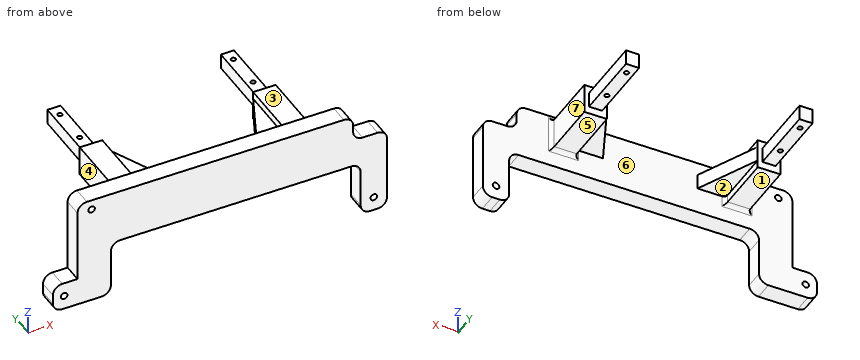
```python
from build123d import *

# Parameters (mm, degrees)
SKETCH1_R           = 1.75
BOSS_EXTRUDE1_DEPTH = 10
SKETCH3_W           = 7
SKETCH3_H           = 8
BOSS_EXTRUDE3_DEPTH = 70
CUT_EXTRUDE1_REACH  = 183.843
SKETCH4_R           = 1.25
SKETCH5_W           = 12
SKETCH5_H           = 16
BOSS_EXTRUDE4_DEPTH = 32.5
FILLET4_R           = 2
RIB1_REACH          = 184.852
SKETCH6_WALL_W      = 403.497752534
SKETCH6_WALL_H      = 8


with BuildPart() as part:
    # Sketch1 → Boss-Extrude1 (new body)
    with BuildSketch(Plane(origin=(0, 0, 0), x_dir=(1, 0, 0), z_dir=(0, 1, 0))):
        with BuildLine():
            Line((-7.5, -0.4), (-7.5, 38.6))
            Line((-7.5, 38.6), (-15.61, 38.6))
            ThreePointArc((-15.61, 38.6), (-19.145533906, 40.064466094), (-20.61, 43.6))
            Line((-20.61, 43.6), (-20.61, 48.6))
            ThreePointArc((-20.61, 48.6), (-19.145533906, 52.135533906), (-15.61, 53.6))
            Line((-15.61, 53.6), (5.26, 53.6))
            ThreePointArc((5.26, 53.6), (8.795533906, 52.135533906), (10.26, 48.6))
            Line((10.26, 48.6), (10.26, 28.6))
            ThreePointArc((10.26, 28.6), (11.724466094, 25.064466094), (15.26, 23.6))
            Line((15.26, 23.6), (138.26, 23.6))
            ThreePointArc((138.26, 23.6), (141.795533906, 25.064466094), (143.26, 28.6))
            Line((143.26, 28.6), (143.26, 48.6))
            ThreePointArc((143.26, 48.6), (144.724466094, 52.135533906), (148.26, 53.6))
            Line((148.26, 53.6), (152.26, 53.6))
            ThreePointArc((152.26, 53.6), (155.795533906, 52.135533906), (157.26, 48.6))
            Line((157.26, 48.6), (157.26, 13.6))
            ThreePointArc((157.26, 13.6), (155.795533906, 10.064466094), (152.26, 8.6))
            Line((152.26, 8.6), (144.26, 8.6))
            ThreePointArc((144.26, 8.6), (140.724466094, 7.135533906), (139.26, 3.6))
            Line((139.26, 3.6), (139.26, -0.4))
            ThreePointArc((139.26, -0.4), (137.795533906, -3.935533906), (134.26, -5.4))
            Line((134.26, -5.4), (-2.5, -5.4))
            ThreePointArc((-2.5, -5.4), (-6.035533906, -3.935533906), (-7.5, -0.4))
        make_face()
        with Locations(Location((0, 0, 0), (0, 0, 270))):
            Circle(SKETCH1_R, mode=Mode.SUBTRACT)
        with Locations(Location((-14.61, 46.1, 0), (0, 0, 270))):
            Circle(SKETCH1_R, mode=Mode.SUBTRACT)
        with Locations(Location((150.26, 46.1, 0), (0, 0, 270))):
            Circle(SKETCH1_R, mode=Mode.SUBTRACT)
    extrude(amount=BOSS_EXTRUDE1_DEPTH)

    # Sketch3 → Boss-Extrude3 (add)
    with BuildSketch(Plane(origin=(0, 10, 0), x_dir=(1, 0, 0), z_dir=(0, 1, 0))):
        with Locations((22, 5.6)):
            Rectangle(SKETCH3_W, SKETCH3_H)
        with Locations((114.32, 5.6)):
            Rectangle(SKETCH3_W, SKETCH3_H)
    extrude(amount=BOSS_EXTRUDE3_DEPTH)

    # Sketch4 → Cut-Extrude1 (cut, up to next)
    with BuildSketch(Plane(origin=(0, 0, -9.6), x_dir=(-1, 0, 0), z_dir=(0, 0, -1)), mode=Mode.PRIVATE) as cut_extrude1_sk1:
        with Locations((-22, 74)):
            Circle(SKETCH4_R)
    cut_extrude1_tool1 = extrude(cut_extrude1_sk1.sketch, amount=-CUT_EXTRUDE1_REACH, mode=Mode.PRIVATE) & part.part
    # Sketch4 → Cut-Extrude1 (cut, up to next)
    with BuildSketch(Plane(origin=(0, 0, -9.6), x_dir=(-1, 0, 0), z_dir=(0, 0, -1)), mode=Mode.PRIVATE) as cut_extrude1_sk2:
        with Locations((-22, 54)):
            Circle(SKETCH4_R)
    cut_extrude1_tool2 = extrude(cut_extrude1_sk2.sketch, amount=-CUT_EXTRUDE1_REACH, mode=Mode.PRIVATE) & part.part
    # Sketch4 → Cut-Extrude1 (cut, up to next)
    with BuildSketch(Plane(origin=(0, 0, -9.6), x_dir=(-1, 0, 0), z_dir=(0, 0, -1)), mode=Mode.PRIVATE) as cut_extrude1_sk3:
        with Locations((-114.32, 54)):
            Circle(SKETCH4_R)
    cut_extrude1_tool3 = extrude(cut_extrude1_sk3.sketch, amount=-CUT_EXTRUDE1_REACH, mode=Mode.PRIVATE) & part.part
    # Sketch4 → Cut-Extrude1 (cut, up to next)
    with BuildSketch(Plane(origin=(0, 0, -9.6), x_dir=(-1, 0, 0), z_dir=(0, 0, -1)), mode=Mode.PRIVATE) as cut_extrude1_sk4:
        with Locations((-114.32, 74)):
            Circle(SKETCH4_R)
    cut_extrude1_tool4 = extrude(cut_extrude1_sk4.sketch, amount=-CUT_EXTRUDE1_REACH, mode=Mode.PRIVATE) & part.part
    add(cut_extrude1_tool1.solids().sort_by_distance((22, 74, -9.6))[0], mode=Mode.SUBTRACT)
    add(cut_extrude1_tool2.solids().sort_by_distance((22, 54, -9.6))[0], mode=Mode.SUBTRACT)
    add(cut_extrude1_tool3.solids().sort_by_distance((114.32, 54, -9.6))[0], mode=Mode.SUBTRACT)
    add(cut_extrude1_tool4.solids().sort_by_distance((114.32, 74, -9.6))[0], mode=Mode.SUBTRACT)

    # Sketch5 → Boss-Extrude4 (add)
    with BuildSketch(Plane(origin=(0, 10, 0), x_dir=(1, 0, 0), z_dir=(0, 1, 0))):
        with Locations((22, 5.6)):
            Rectangle(SKETCH5_W, SKETCH5_H)
        with Locations((114.32, 5.6)):
            Rectangle(SKETCH5_W, SKETCH5_H)
    extrude(amount=BOSS_EXTRUDE4_DEPTH)

    # Fillet4
    fillet4_edges = [part.edges().sort_by_distance(p)[0] for p in [
        (16, 10, -5.6),
        (22, 10, 2.4),
        (28, 10, -5.6),
        (22, 10, -13.6),
        (108.32, 10, -5.6),
        (114.32, 10, 2.4),
        (120.32, 10, -5.6),
        (114.32, 10, -13.6),
    ]]
    fillet(fillet4_edges, radius=FILLET4_R)

    # Sketch6 wall → Rib1 (add, up to next)
    with BuildSketch(Plane(origin=(100.82, 26.25, -5.6), x_dir=(-0.419058177462, -0.9079593845, 0), z_dir=(-0.9079593845, 0.419058177462, 0)), mode=Mode.PRIVATE) as rib1_sk1:
        Rectangle(SKETCH6_WALL_W, SKETCH6_WALL_H)
    rib1_tool1 = extrude(rib1_sk1.sketch, amount=-RIB1_REACH, mode=Mode.PRIVATE) - part.part
    rib1 = rib1_tool1.solids().sort_by_distance((100.82, 26.25, -5.6))[0]
    add(rib1)

    # Mirror1: Rib1 across plane
    add(rib1.mirror(Plane(origin=(68.16, 0, 0), x_dir=(0, 0, 1), z_dir=(1, 0, 0))))


solid = part.part
```
Check sheet for the modelled part. Datum: model origin and axes. Units: mm. Face numbers are marked on the shaded views. A direction names the side the tool comes from. Give positions to 0.01 mm unless a question says otherwise; leave off trailing zeros. Order: outer loops, then holes, each group sorted by start corner. A loop starts at its lowest first (then second) coordinate and runs counter-clockwise, first axis right, second up. Notation, with made-up numbers: (48, 68) -> (71, 68) arc R12 cw to (71, 82) -> close; hole circle Ø9 at (43, -37.5). An arc over 180 degrees is marked (long way). Return JSON: item names as keys, results as strings.
1. Material ranges on probe 1 along Y at (x, z) = (114, -5); probe 2 along X at (y, z) = (6.5, -46.1); probe 3 along X at (y, z) = (58, -5), recorded low to high. Write a range as [from, to].
From the geometry:
{"probe 1": "[0, 52.79], [55.21, 72.79], [75.21, 80]", "probe 2": "[-20.61, -16.36], [-12.86, 10.26], [143.26, 148.51], [152.01, 157.26]", "probe 3": "[18.5, 25.5], [110.82, 117.82]"}
2. Go/stop test with flat-tipped pins: P1, Ø3.5, axis at x = 112.5, y = 68, coming from the +Z side; P2, Ø8, axis at x = 50.5, z = -11.5, coming from the +Y side; P3, Ø4, axis at y = 56, z = -6.5, coming from the -X side; P4, Ø12, axis at x = 100.5, y = 57, coming from the -Z side. Record where each tip stops, or that it passes through.
From the geometry:
{"P1": "z = -1.6", "P2": "y = 10", "P3": "x = 18.5", "P4": "through"}
3. Cross-section at A-A, the plane z = -35.5. Record the cut outline in (x, y).
From the geometry:
{"outline": "(-7.5, 0) -> (10.26, 0) -> (10.26, 10) -> (-7.5, 10) -> close; (143.26, 0) -> (157.26, 0) -> (157.26, 10) -> (143.26, 10) -> close"}
4. Cross-section at B-B, the plane y = 64.5. Record the cut outline in (x, z).
From the geometry:
{"outline": "(18.5, -9.6) -> (25.5, -9.6) -> (25.5, -1.6) -> (18.5, -1.6) -> close; (110.82, -9.6) -> (117.82, -9.6) -> (117.82, -1.6) -> (110.82, -1.6) -> close"}
5. Set-up check for the marked faces 1, 2, 3 and 4: record each of +Z, -Z, +X, -X, +Y, -Y from which the full face is reachable in a straight line by a thin tool's end or side.
From the geometry:
{"face 1": "-Z, +X, -X, +Y", "face 2": "-Z, +Y", "face 3": "+Z, +X, -X, +Y", "face 4": "+Z, -Z, -X, +Y"}
6. Cross-section at C-C, the plane z = -46.1. Record the cut outline in (x, y), plus the area to 3 significant figures.
From the geometry:
{"outline": "(-20.61, 0) -> (-16.36, 0) -> (-16.36, 10) -> (-20.61, 10) -> close; (-12.86, 0) -> (10.26, 0) -> (10.26, 10) -> (-12.86, 10) -> close; (143.26, 0) -> (148.51, 0) -> (148.51, 10) -> (143.26, 10) -> close; (152.01, 0) -> (157.26, 0) -> (157.26, 10) -> (152.01, 10) -> close", "area": "379 mm^2"}
7. Mould release check, pull along X, two halves, no side actions. Record for the marked faces 5, 6 and 7: +X half, -X half, draft (parallel to the pull), parting line (faces both ways), or undercut.
From the geometry:
{"face 5": "draft", "face 6": "undercut", "face 7": "+X half"}
8. Cross-section at D-D, the plane x = 41. Record the cut outline in (y, z).
From the geometry:
{"outline": "(0, -23.6) -> (10, -23.6) -> (10, -9.6) -> (14.33, -9.6) -> (14.33, -1.6) -> (10, -1.6) -> (10, 5.4) -> (0, 5.4) -> close"}
